Check sheet for the modelled part. Datum: model origin and axes. Units: mm. Coordinates: 2 decimals unless noted, no trailing zeros.
1. Gauge pin test, flat end, axial feed: pin 1 Ø2 at (x, z) = (4.5, -28) entering from -Y. Record the tip position at first contact, or that the pin passes through.
2. Cross-section at B-B (y = 0.55). Count the separate pieces of the cut face and the enclosed holes in it, then the cut area to 3 significant figures.
3. Thickness scan on line 1 (X direction, y = 1.75, z = 0); line 2 (X direction, y = 0.8, z = 0); line 3 (X direction, y = 1, z = 40). Record the ranges inside material, lowest first.
```python
from build123d import *

# Parameters (mm, degrees)
SKETCH1_R           = 45
BOSS_EXTRUDE1_DEPTH = 3
SKETCH2_R           = 1.75
CUT_EXTRUDE1_DEPTH  = 10
SKETCH3_R           = 10
CUT_EXTRUDE2_DEPTH  = 5
FILLET1_R           = 1.5
FILLET2_R           = 1.5


with BuildPart() as part:
    # Sketch1 → Boss-Extrude1 (new body)
    with BuildSketch(Plane(origin=(0, 0, 0), x_dir=(1, 0, 0), z_dir=(0, 1, 0))):
        with Locations(Location((0, 0, 0), (0, 0, 270))):
            Circle(SKETCH1_R)
    extrude(amount=BOSS_EXTRUDE1_DEPTH)

    # Sketch2 → Cut-Extrude1 (cut)
    with BuildSketch(Plane(origin=(0, 3, 0), x_dir=(1, 0, 0), z_dir=(0, 1, 0))):
        with Locations(Location((-5, -40, 0), (0, 0, 270))):
            Circle(SKETCH2_R)
        with Locations(Location((5, -40, 0), (0, 0, 270))):
            Circle(SKETCH2_R)
        with Locations(Location((-5, 40, 0), (0, 0, 270))):
            Circle(SKETCH2_R)
        with Locations(Location((5, 40, 0), (0, 0, 270))):
            Circle(SKETCH2_R)
        with Locations(Location((-40, 0, 0), (0, 0, 270))):
            Circle(SKETCH2_R)
        with Locations(Location((40, 0, 0), (0, 0, 270))):
            Circle(SKETCH2_R)
        with Locations(Location((-5, -15, 0), (0, 0, 270))):
            Circle(SKETCH2_R)
        with Locations(Location((5, 15, 0), (0, 0, 270))):
            Circle(SKETCH2_R)
    extrude(amount=-CUT_EXTRUDE1_DEPTH, mode=Mode.SUBTRACT)

    # Sketch3 → Cut-Extrude2 (cut)
    with BuildSketch(Plane(origin=(0, 3, 0), x_dir=(1, 0, 0), z_dir=(0, 1, 0))):
        with Locations(Location((0, 0, 0), (0, 0, 270))):
            Circle(SKETCH3_R)
    extrude(amount=-CUT_EXTRUDE2_DEPTH, mode=Mode.SUBTRACT)

    # Fillet1
    fillet1_edges = [part.edges().sort_by_distance(p)[0] for p in [
        (0, 0, -45),
        (0, 3, -45),
    ]]
    fillet(fillet1_edges, radius=FILLET1_R - 0.0001)  # a hair under: the kernel refuses the full size

    # Fillet2
    fillet2_edges = [part.edges().sort_by_distance(p)[0] for p in [
        (0, 0, -10),
        (0, 3, -10),
    ]]
    fillet(fillet2_edges, radius=FILLET2_R - 0.0001)  # a hair under: the kernel refuses the full size


solid = part.part
```
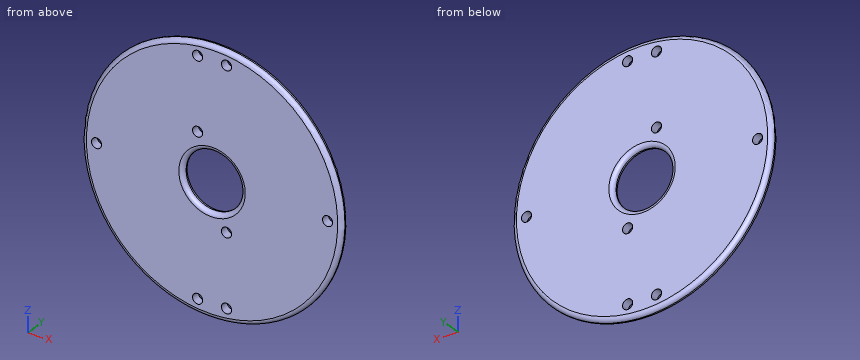
Data:
1. pin 1: stops at y = 0
2. separate pieces: 1
2. enclosed holes: 9
2. area: 5,850 mm2
3. line 1: x = -44.98 to -41.75, -38.25 to -10.02, 10.02 to 38.25, 41.75 to 44.98
3. line 2: x = -44.83 to -41.75, -38.25 to -10.17, 10.17 to 38.25, 41.75 to 44.83
3. line 3: x = -20.43 to -6.75, -3.25 to 3.25, 6.75 to 20.43
